Check sheet for the modelled part. Datum: model origin and axes. Units: mm. A direction names the side the tool comes from. Round coordinates to 2 decimals unless told otherwise and drop trailing zeros. Order: outer loops, then holes, each group sorted by start corner. A loop starts at its lowest first (then second) coordinate and runs counter-clockwise, first axis right, second up.
Q1. Cross-section at D-D on z = 170. Record the cut outline in (x, y), then the cut area to 3 significant figures.
Q2. Mould release check, pull along X, two halves, no side actions. Record for faces 5 (the flat face through (182, 63, 352)), 6 (the flat face through (78, -4, 352)), 7 (the cylindrical face through (-185.944, -59.632, 545.518)): +X half, -X half, draft (parallel to the pull), parting line (faces both ways), or undercut.
Q3. Cross-section at B-B on x = 0. Record the cut outline in (y, z).
Q4. Scan lines: probe 1 along Y at (x, z) = (-187.25, 170); probe 2 along X at (y, z) = (-9.5, 395.5); probe 3 along Y at (x, z) = (-141.5, 186.5). Record each from-to range of solid material in increasing order.
Q5. Depth check by flat-ended pin: P1, Ø1.5, axis at x = -111, z = 548, coming from the -Y side; P2, Ø2, axis at x = 66, z = 370, coming from the +Y side. Enter the tip coordinate at first touch or a pass-through.
Q6. Cross-section at A-A on z = 402. Record the cut outline in (x, y).
Q7. Cross-section at C-C on y = -103.5. Record the cut outline in (x, z).
Q8. Set-up check for faces 1 (the cylindrical face through (186.056, -70.344, 648.716)), 2 (the cylindrical face through (-1.319, 0.056, 196.765)), 3 (the flat face through (-78, 4, 352)), 4 (the flat face through (182, -61, 352)): record each of +Z, -Z, +X, -X, +Y, -Y from which the full face is reachable in a straight line by a thin tool's end or side.
from build123d import *

# Parameters (mm, degrees)
EXTRUDE_1_DEPTH     = 713.5
SKETCH_2_R          = 15.5
CUT_EXTRUDE_2_DEPTH = 818.240631638
CUT_EXTRUDE_3_DEPTH = 749.704380914


with BuildPart() as part:
    # 草图1 → 拉伸1 (new body)
    with BuildSketch(Plane.XY):
        Polygon((-182, 120), (-190, 120), (-190, -120), (-182, -120), (-182, -4), (182, -4), (182, -120), (190, -120), (190, 120), (182, 120), (182, 4), (-182, 4), align=None)
    extrude(amount=EXTRUDE_1_DEPTH)

    # 草图2 → 拉伸2 (cut, through all)
    with BuildSketch(Plane(origin=(190, 0, 0), x_dir=(0, 0, -1), z_dir=(1, 0, 0))):
        with Locations((-663.5, 75)):
            Circle(SKETCH_2_R)
        with Locations((-543.5, 75)):
            Circle(SKETCH_2_R)
        with Locations((-663.5, -75)):
            Circle(SKETCH_2_R)
        with Locations((-543.5, -75)):
            Circle(SKETCH_2_R)
        with Locations((-170, 75)):
            Circle(SKETCH_2_R)
        with Locations((-50, 75)):
            Circle(SKETCH_2_R)
        with Locations((-50, -75)):
            Circle(SKETCH_2_R)
        with Locations((-170, -75)):
            Circle(SKETCH_2_R)
        Polygon((-673.5, 120), (-713.5, 80), (-713.5, 120), align=None)
        Polygon((-40, 120), (0, 80), (0, 120), align=None)
        Polygon((-40, -120), (0, -80), (0, -120), align=None)
        Polygon((-673.5, -120), (-713.5, -80), (-713.5, -120), align=None)
    extrude(amount=-CUT_EXTRUDE_2_DEPTH, mode=Mode.SUBTRACT)

    # 草图3 → 拉伸3 (cut, through all)
    with BuildSketch(Plane(origin=(0, 4, 0), x_dir=(1, 0, 0), z_dir=(0, 1, 0))):
        with BuildLine():
            Line((60, -256.75), (60, -456.75))
            ThreePointArc((60, -456.75), (0, -516.75), (-60, -456.75))
            Line((-60, -456.75), (-60, -256.75))
            ThreePointArc((-60, -256.75), (0, -196.75), (60, -256.75))
        make_face()
    extrude(amount=-CUT_EXTRUDE_3_DEPTH, mode=Mode.SUBTRACT)


solid = part.part
Results found:
1. outline: (-190, -120) - (-182, -120) - (-182, -90.5) - (-190, -90.5) - close; (-190, -59.5) - (-182, -59.5) - (-182, -4) - (182, -4) - (182, -59.5) - (190, -59.5) - (190, 59.5) - (182, 59.5) - (182, 4) - (-182, 4) - (-182, 59.5) - (-190, 59.5) - close; (-190, 90.5) - (-182, 90.5) - (-182, 120) - (-190, 120) - close; (182, -120) - (190, -120) - (190, -90.5) - (182, -90.5) - close; (182, 90.5) - (190, 90.5) - (190, 120) - (182, 120) - close
1. area: 5,760 mm2
2. face 5: undercut
2. face 6: undercut
2. face 7: draft
3. outline: (-4, 0) - (4, 0) - (4, 196.75) - (-4, 196.75) - close; (-4, 516.75) - (4, 516.75) - (4, 713.5) - (-4, 713.5) - close
4. probe 1: y = -120 to -90.5, -59.5 to 59.5, 90.5 to 120
4. probe 2: x = -190 to -182, 182 to 190
4. probe 3: y = -4 to 4
5. P1: stops at y = -4
5. P2: stops at y = 4
6. outline: (-190, -120) - (-182, -120) - (-182, -4) - (-60, -4) - (-60, 4) - (-182, 4) - (-182, 120) - (-190, 120) - close; (60, -4) - (182, -4) - (182, -120) - (190, -120) - (190, 120) - (182, 120) - (182, 4) - (60, 4) - close
7. outline: (-190, 23.5) - (-182, 23.5) - (-182, 690) - (-190, 690) - close; (182, 23.5) - (190, 23.5) - (190, 690) - (182, 690) - close
8. face 1: +X, -X
8. face 2: +Y, -Y
8. face 3: +Z, -Z, +Y
8. face 4: +Z, -Z, -Y
